Autodesk Fusion 360 part; units mm, degrees
sketch "Boceto1" plane through (0, 0, 0) normal (0, 0, 1) x (1, 0, 0)
  line L0 (0, 0) -> (230, 0)
  line L1 (230, 0) -> (230, 165)
  line L2 (230, 165) -> (0, 165)
  line L3 (0, 165) -> (0, 0)
  line L4 (0, 165) -> (25, 165)
  line L5 (25, 165) -> (25, 140)
  line L6 (25, 140) -> (0, 140)
  line L7 (0, 140) -> (0, 165)
  line L8 (230, 165) -> (205, 165)
  line L9 (205, 165) -> (205, 140)
  line L10 (205, 140) -> (230, 140)
  line L11 (230, 140) -> (230, 165)
  line L12 (230, 0) -> (205, 0)
  line L13 (205, 0) -> (205, 25)
  line L14 (205, 25) -> (230, 25)
  line L15 (230, 25) -> (230, 0)
  line L16 (0, 0) -> (25, 0)
  line L17 (25, 0) -> (25, 25)
  line L18 (25, 25) -> (0, 25)
  line L19 (0, 25) -> (0, 0)
  dimension "d1" = 230
  dimension "d2" = 165
  dimension "d12" = 25
ref_plane "WorkPlane1" through (115, 82.5, 83) normal (0, 0, 1) x (1, 0, 0)
extrude "Extrude4" add sketch "Boceto1" along normal blind 83 contours L0 L3 L16 L17 L18 L19 | L0 L1 L12 L13 L14 L15 | L2 L3 L4 L5 L6 L7 | L1 L2 L8 L9 L10 L11 makes body 1 at (0, 16.6667, 27.6667) makes body 2 at (205, 8.3333, 27.6667) makes body 3 at (0, 156.6667, 27.6667) makes body 4 at (213.3333, 140, 27.6667)
sketch "Sketch4" plane through (0, 0, 83) normal (0, 0, 1) x (1, 0, 0)
  line L0 (25, 25) -> (0, 25)
  line L1 (25, 0) -> (25, 25)
  line L2 (0, 0) -> (25, 0)
  line L3 (0, 25) -> (0, 0)
  line L4 (0, 140) -> (0, 165)
  line L5 (0, 165) -> (25, 165)
  line L6 (25, 165) -> (25, 140)
  line L7 (25, 140) -> (0, 140)
  line L8 (205, 140) -> (230, 140)
  line L9 (205, 165) -> (205, 140)
  line L10 (230, 165) -> (205, 165)
  line L11 (230, 140) -> (230, 165)
  line L12 (230, 25) -> (230, 0)
  line L13 (230, 0) -> (205, 0)
  line L14 (205, 0) -> (205, 25)
  line L15 (205, 25) -> (230, 25)
  line L16 (0, 0) -> (230, 0)
  line L17 (230, 0) -> (230, 165)
  line L18 (230, 165) -> (0, 165)
  line L19 (0, 165) -> (0, 0)
extrude "Extrude5" add sketch "Sketch4" against normal blind 15 bodies 1 2 3 4
sketch "Sketch5" plane through (0, 0, 83) normal (0, 0, 1) x (-1, 0, 0)
  line L0 (-230, -165) -> (0, -165)
  line L1 (0, -165) -> (0, 0)
  line L2 (0, 0) -> (-230, 0)
  line L3 (-230, 0) -> (-230, -165)
  line L4 (-5, -5) -> (-225, -5)
  line L5 (-225, -5) -> (-225, -160)
  line L6 (-225, -160) -> (-5, -160)
  line L7 (-5, -160) -> (-5, -5)
  dimension "d17" = -5
fillet "Fillet1" radius 25 8 edges at (12.5, 25, 68) (25, 12.5, 68) (25, 152.5, 68) (12.5, 140, 68) (217.5, 140, 68) (205, 152.5, 68) (205, 12.5, 68) (217.5, 25, 68) on bodies 1
fillet "Fillet2" radius 5 20 edges at (205, 0, 21.5) (197.6777, 0, 60.6777) (115, 0, 68) (32.3223, 0, 60.6777) (25, 0, 21.5) (230, 140, 21.5) (230, 132.6777, 60.6777) (230, 82.5, 68) (230, 32.3223, 60.6777) (230, 25, 21.5) (25, 165, 21.5) (32.3223, 165, 60.6777) (115, 165, 68) (197.6777, 165, 60.6777) (205, 165, 21.5) (0, 25, 21.5) (0, 32.3223, 60.6777) (0, 82.5, 68) (0, 132.6777, 60.6777) (0, 140, 21.5) on bodies 1
fillet "Fillet3" radius 2 8 edges at (0, 82.5, 83) (115, 0, 83) (0, 0, 41.5) (230, 0, 41.5) (230, 82.5, 83) (230, 165, 41.5) (115, 165, 83) (0, 165, 41.5) on bodies 1
CAD build for the part. Positions are in the model's coordinates, mm. A direction names the side the tool comes from. Coordinates: 2 decimals unless noted, no trailing zeros. Loops run counter-clockwise (first coordinate to the right, second up) from the corner with the lowest first, then second, coordinate; pieces in that order, holes last. Notation, with made-up numbers: (-16, 8) - (14, 8) arc R21 ccw to (14, 17) - close; hole circle Ø3 at (39.5, 19). An arc over 180 degrees is marked (long way). Use one line per item in the form item = value. Start each with the question number.
1) Band-saw the part on A-A (z = 14). Give the cut face in (x, y), and give its area (3 significant figures).
2) Drill centre lines: L1, parallel to X at y = 150.5, z = 18; L2, parallel to Z at x = 72.5, y = 73; L3, parallel to Y at x = 216.5, z = 3. Where is each one in solid material? Low to high. Write a range as from..to.
3) Flat gauge pins, fed straight in: pin 1 (10 mm diameter, centred on x = 212.5, z = 11, fed in from -Y); pin 2 (4 mm diameter, centred on x = 77, y = 110.5, fed in from -Z). Where does each tip first touch, or does it go through?
4) Tool access for faces 4 (the face through (207.815, 35.887, 63.635)), 5 (the face through (206, 2, 22)), 6 (the face through (195, 142, 63)), 7 (the face through (2, 141, 21)): list every direction of +Z, -Z, +X, -X, +Y, -Y with a clear straight run to the whole face (end or side of a thin tool).
5) Band-saw the part on C-C (x = 149). Give the cut face in (y, z), and give its area (3 significant figures).
6) Band-saw the part on D-D (z = 50). State how many separate pieces and enclosed holes the cut face has, and give its area (3 significant figures).
7) Band-saw the part on B-B (y = 93). Give the cut face in (x, z), and give its area (3 significant figures).
8) Two-plate mould, pull along Y, no slides. Class faces 1 (the face through (106.1, 0, 73.3)), 2 (the face through (215, 25, 21)), 3 (the face through (217, 153, 0)): +Y half, -Y half, draft (parallel to the pull), parting line (faces both ways), or undercut.
Check values:
q1.outline = (0, 2) arc R2 ccw to (2, 0) - (20, 0) arc R5 ccw to (25, 5) - (25, 25) - (5, 25) arc R5 ccw to (0, 20) - close; (0, 145) arc R5 ccw to (5, 140) - (25, 140) - (25, 160) arc R5 ccw to (20, 165) - (2, 165) arc R2 ccw to (0, 163) - close; (205, 5) arc R5 ccw to (210, 0) - (228, 0) arc R2 ccw to (230, 2) - (230, 20) arc R5 ccw to (225, 25) - (205, 25) - close; (205, 140) - (225, 140) arc R5 ccw to (230, 145) - (230, 163) arc R2 ccw to (228, 165) - (210, 165) arc R5 ccw to (205, 160) - close
q1.area = 2,450 mm2
q2.L1 = 0..25, 205..230
q2.L2 = 68..83
q2.L3 = 0..25, 140..165
q3.pin_1 = 0
q3.pin_2 = 68
q4.face_4 = -Z, +X, -X
q4.face_5 = -Z, -Y
q4.face_6 = -Z, +Y, -Y
q4.face_7 = -Z, -X
q5.outline = (0, 73) arc R5 ccw to (5, 68) - (160, 68) arc R5 ccw to (165, 73) - (165, 81) arc R2 ccw to (163, 83) - (2, 83) arc R2 ccw to (0, 81) - close
q5.area = 2,460 mm2
q6.separate_pieces = 4
q6.enclosed_holes = 0
q6.area = 2,660 mm2
q7.outline = (0, 73) arc R5 ccw to (5, 68) - (225, 68) arc R5 ccw to (230, 73) - (230, 81) arc R2 ccw to (228, 83) - (2, 83) arc R2 ccw to (0, 81) - close
q7.area = 3,440 mm2
q8.face_1 = -Y half
q8.face_2 = undercut
q8.face_3 = draft
